```python
from build123d import *

# Parameters (mm, degrees)
ESBO_O1_R                = 3.5
RESSALTO_EXTRUS_O1_DEPTH = 5
RESSALTO_EXTRUS_O2_DEPTH = 1.4
ESBO_O3_R                = 0.5
CORTE_EXTRUS_O1_DEPTH    = 18.12454379
PADR_O_LINEAR1_COUNT     = 6
PADR_O_LINEAR1_PITCH     = 2


with BuildPart() as part:
    # Esbo_o1 → Ressalto-extrus_o1 (new body)
    with BuildSketch(Plane(origin=(0, 0, 0), x_dir=(1, 0, 0), z_dir=(0, 1, 0))):
        with Locations(Location((0, 0, 0), (0, 0, 270))):
            Circle(ESBO_O1_R)
    extrude(amount=RESSALTO_EXTRUS_O1_DEPTH)

    # Esbo_o2 → Ressalto-extrus_o2 (add)
    with BuildSketch(Plane(origin=(0, 0, 0), x_dir=(1, 0, 0), z_dir=(0, 1, 0))):
        with BuildLine():
            Line((-14.214285714, 1.988487272), (-0.375, 3.479852727))
            Line((-0.375, 3.479852727), (-0.375, -3.479852727))
            Line((-0.375, -3.479852727), (-14.214285714, -1.988487272))
            ThreePointArc((-14.214285714, -1.988487272), (-16, 0), (-14.214285714, 1.988487272))
        make_face()
    extrude(amount=RESSALTO_EXTRUS_O2_DEPTH)

    # Esbo_o3 → Corte-extrus_o1 (cut, through all)
    with BuildSketch(Plane(origin=(0, 0, 0), x_dir=(1, 0, 0), z_dir=(0, 1, 0))):
        with Locations(Location((-14.7, 0, 0), (0, 0, 270))):
            Circle(ESBO_O3_R)
    corte_extrus_o1 = extrude(amount=CORTE_EXTRUS_O1_DEPTH, mode=Mode.SUBTRACT)

    # Padr_o linear1: Corte-extrus_o1 ×6
    with Locations(*[(i * PADR_O_LINEAR1_PITCH, 0, 0) for i in range(1, PADR_O_LINEAR1_COUNT)]):
        add(corte_extrus_o1, mode=Mode.SUBTRACT)


solid = part.part
```
Check sheet for the modelled part. Datum: model origin and axes. Units: mm. A direction names the side the tool comes from. Round coordinates to 2 decimals unless told otherwise and drop trailing zeros. Loops run counter-clockwise (first coordinate to the right, second up) from the corner with the lowest first, then second, coordinate; pieces in that order, holes last. Notation, with made-up numbers: (-14.75, 46.25) - (41.25, 46.25) arc R21 ccw to (41.25, 70.25) - close; hole circle Ø2 at (56, 32.5). An arc over 180 degrees is marked (long way). Answer as a JSON object with one key per item and string values. Group by question number.
Q1. Scan lines: line 1 along Y through (x, z) = (-10.5, 1.25); line 2 along Z through (x, y) = (-12.7, 0.4); line 3 along Z through (x, y) = (-10.7, 0.8). Record each from-to range of solid material in increasing order. Write a range as [from, to].
Q2. Sectioned sample at C-C, the plane x = -4.5. Enter the section's corners in (y, z).
Q3. Sectioned sample at B-B, the plane z = 0. Count the separate pieces of the cut face and the enclosed holes in it, plus the area to 3 significant figures.
Q4. Sectioned sample at A-A, the plane y = 1. Enter the section's corners in (x, z) (3 decimals).
Q5. Sectioned sample at D-D, the plane x = -14.7. Enter the section's corners in (y, z).
Q6. Set-up check for faces 1 (the face through (3.47, 3.02, -0.46)), 2 (the face through (-13.144, 0.69, 0.231)): record each of +Z, -Z, +X, -X, +Y, -Y from which the full face is reachable in a straight line by a thin tool's end or side.
Q7. Gauge pin test, flat ends, axial feed: P1, Ø1, axis at x = -11, z = 2.5, coming from the -Y side; P2, Ø3, axis at x = -6.5, y = 1, coming from the -Z side; P3, Ø3, axis at x = -11.5, z = 2, coming from the +Y side. Record the tip position at first contact, or that the pin passes through.
Solution:
{
 "1": {"line 1": "y = [0, 1.4]", "line 2": "z = [-2.15, -0.5], [0.5, 2.15]", "line 3": "z = [-2.37, -0.5], [0.5, 2.37]"},
 "2": {"outline": "(0, -3.04) - (1.4, -3.04) - (1.4, -0.46) - (0, -0.46) - close; (0, 0.46) - (1.4, 0.46) - (1.4, 3.04) - (0, 3.04) - close"},
 "3": {"separate pieces": "7", "enclosed holes": "0", "area": "44.1 mm²"},
 "4": {"outline": "(-14.214, -1.988) - (-0.375, -3.48) arc R3.5 ccw (long way) to (-0.375, 3.48) - (-14.214, 1.988) arc R2 ccw to start; hole circle Ø1 at (-14.7, 0); hole circle Ø1 at (-12.7, 0); hole circle Ø1 at (-10.7, 0); hole circle Ø1 at (-8.7, 0); hole circle Ø1 at (-6.7, 0); hole circle Ø1 at (-4.7, 0)"},
 "5": {"outline": "(0, -1.87) - (1.4, -1.87) - (1.4, -0.5) - (0, -0.5) - close; (0, 0.5) - (1.4, 0.5) - (1.4, 1.87) - (0, 1.87) - close"},
 "6": {"face 1": "+Y", "face 2": "+Y, -Y"},
 "7": {"P1": "stops at y = 0", "P2": "stops at z = -2.98", "P3": "stops at y = 1.4"}
}
